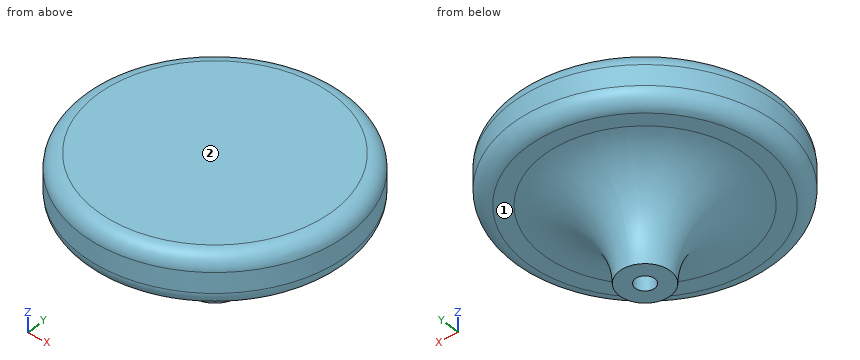
from build123d import *

# Parameters (mm, degrees)
SKETCH1_R           = 4.233333333
BOSS_EXTRUDE1_DEPTH = 12.7
SKETCH2_R           = 22.225
BOSS_EXTRUDE3_DEPTH = 8.466666667
FILLET1_R           = 12.7
FILLET2_R           = 2.54
SKETCH5_R           = 1.6256
CUT_EXTRUDE2_DEPTH  = 15.621


with BuildPart() as part:
    # Sketch1 → Boss-Extrude1 (new body)
    with BuildSketch(Plane.XY):
        Circle(SKETCH1_R)
    extrude(amount=BOSS_EXTRUDE1_DEPTH)

    # Sketch2 → Boss-Extrude3 (add)
    with BuildSketch(Plane.XY.offset(12.7)):
        Circle(SKETCH2_R)
    extrude(amount=BOSS_EXTRUDE3_DEPTH)

    # Fillet1
    fillet1_edges = [part.edges().sort_by_distance(p)[0] for p in [
        (-4.233333333, 0, 12.7),
    ]]
    fillet(fillet1_edges, radius=FILLET1_R - 0.0001)  # a hair under: the kernel refuses the full size

    # Fillet2
    fillet2_edges = [part.edges().sort_by_distance(p)[0] for p in [
        (-22.225, 0, 12.7),
        (-22.225, 0, 21.166666667),
    ]]
    fillet(fillet2_edges, radius=FILLET2_R)

    # Sketch5 → Cut-Extrude2 (cut)
    with BuildSketch(Plane(origin=(0, 0, 0), x_dir=(-1, 0, 0), z_dir=(0, 0, -1))):
        Circle(SKETCH5_R)
    extrude(amount=-CUT_EXTRUDE2_DEPTH, mode=Mode.SUBTRACT)


solid = part.part
Design review of the part built by this model. Coordinates are the model's own, in mm. Face numbers are marked on the shaded views. A direction names the side the tool comes from. Round coordinates to 2 decimals unless told otherwise and drop trailing zeros. Loops run counter-clockwise (first coordinate to the right, second up) from the corner with the lowest first, then second, coordinate; pieces in that order, holes last. Notation, with made-up numbers: (0, 21) - (31, 21) arc R19 ccw to (31, 56) - close; hole circle Ø4 at (55, 62). An arc over 180 degrees is marked (long way). One line per question, with ' | ' between items.
1. For L1, parallel to Y at x = 0, z = 9.75; L2, parallel to Y at x = 0, z = 7.25; L3, parallel to Z at x = -12, y = -14, list the stretches that pass through material, from the lowest coordinate up. Write a range as [from, to].
Results are:
L1: y = [-8.8, -1.63], [1.63, 8.8] | L2: y = [-6.51, -1.63], [1.63, 6.51] | L3: z = [12.7, 21.17]
2. We need section D-D, the plane z = 3. State the section outline as (x, y) points, and give its area (3 significant figures).
Results are:
outline: circle Ø9.19 at (0, 0); hole circle Ø3.25 at (0, 0) | area: 58.0 mm²
3. For the marked faces 1 and 2, list the 3-axis set-ups (+Z, -Z, +X, -X, +Y, -Y) from which the entire face can be reached by the end or side of a thin tool; tool diameter is ignored.
Results are:
face 1: -Z | face 2: +Z, +X, -X, +Y, -Y
4. Clearance check with flat-ended pins moving along their axes: P1, Ø12, axis at x = 9.5, z = 11, coming from the -Y side; P2, Ø8, axis at x = -17, z = 15.5, coming from the +Y side; P3, Ø4, axis at x = 10.5, z = 18, coming from the +Y side. State where each tip first meets the part, or that it passes through.
Results are:
P1: stops at y = -21.65 | P2: stops at y = 18.03 | P3: stops at y = 20.54
5. We need section C-C, the plane z = 6. State the section outline as (x, y) points.
Results are:
outline: circle Ø11.48 at (0, 0); hole circle Ø3.25 at (0, 0)
